Check sheet for the modelled part. Datum: model origin and axes. Units: mm. Face numbers are marked on the shaded views. A direction names the side the tool comes from. Round coordinates to 2 decimals unless told otherwise and drop trailing zeros. Order: outer loops, then holes, each group sorted by start corner. A loop starts at its lowest first (then second) coordinate and runs counter-clockwise, first axis right, second up. Notation, with made-up numbers: M 20,-37 L 33,-37 A14 cw 33,-20 Z; hole C 38.5,-5.75 d3. An arc over 180 degrees is marked long. One line per item, written item: value. Start each with the question number.
(1) Cross-section at C-C, the plane z = 20. Enter the section's corners in (x, y).
(2) Depth check by flat-ended pin: pin 1 Ø6 at (y, z) = (12, 19) entering from +X; pin 2 Ø5 at (x, y) = (31, 36.5) entering from +Z; pin 3 Ø2.5 at (x, y) = (17, -3.5) entering from -Z. Enter the tip coordinate at first touch or a pass-through.
(3) Cross-section at B-B, the plane y = 22. Enter the section's corners in (x, z), and give its area (3 significant figures).
(4) Cross-section at D-D, the plane y = 50.5. Enter the section's corners in (x, z).
(5) Thickness scan on L1, parallel to Z at x = 22.5, y = 22; L2, parallel to Y at x = 35, z = 33; L3, parallel to X at y = 7, z = 27.5. Record the ranges inside material, lowest first.
(6) Cross-section at A-A, the plane x = 31.5. Enter the section's corners in (y, z).
(7) Access from +Z, -Z, +X, -X, +Y, -Y to the whole of each face (thin tool, end or side, straight path). Record for the marked faces 1, 2 and 3.
from build123d import *

# Parameters (mm, degrees)
F0_W     = 40
F0_H     = 40
F1_DEPTH = 4
F0_H_2   = 6
F2_DEPTH = 48
F3_W     = 40
F3_H     = 3
F4_DEPTH = 5
F6_DEPTH = 3
F7_DEPTH = 20


with BuildPart() as f1:
    # F0 (on Top) → F1 (new body)
    with BuildSketch(Plane.XY):
        with Locations((20, 26)):
            Rectangle(F0_W, F0_H)
    extrude(amount=F1_DEPTH)

    # F0 (on Top) → F2 (join)
    with BuildSketch(Plane.XY):
        with Locations((20, 3)):
            Rectangle(F0_W, F0_H_2)
    extrude(amount=F2_DEPTH)

    # F3 (on face) → F4 (join)
    with BuildSketch(Plane.XZ):
        with Locations((20, 46.5)):
            Rectangle(F3_W, F3_H)
    extrude(amount=F4_DEPTH)

    # F5 (on face) → F6 (join)
    with BuildSketch(Plane(origin=(0, 0, 0), x_dir=(0, -1, 0), z_dir=(-1, 0, 0))):
        Polygon((-6, 48), (-46, 4), (-6, 4), align=None)
    extrude(amount=-F6_DEPTH)

    # F1_face (on face) → F7 (join)
    with BuildSketch(Plane(origin=(20, 46, 2), x_dir=(-1, 0, 0), z_dir=(0, 1, 0))):
        Polygon((-20, 2), (-20, -2), (20, -2), (20, 2), (17, 2), align=None)
    extrude(amount=F7_DEPTH)


solid = f1.part
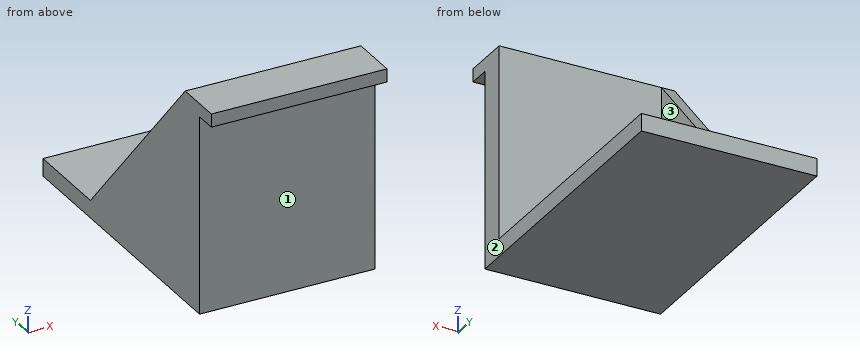
Values found:
1. outline: M 0,0 L 40,0 L 40,6 L 3,6 L 3,31.45 L 0,31.45 Z
2. pin 1: x = 3
2. pin 2: z = 4
2. pin 3: z = 45
3. outline: M 0,0 L 40,0 L 40,4 L 3,4 L 3,30.4 L 0,30.4 Z
3. area: 239 mm^2
4. outline: M 0,0 L 40,0 L 40,4 L 0,4 Z
5. L1: 0 to 4
5. L2: 0 to 6
5. L3: 0 to 3
6. outline: M -5,45 L 0,45 L 0,0 L 66,0 L 66,4 L 6,4 L 6,48 L -5,48 Z
7. face 1: -Z, +X, -X, -Y
7. face 2: +Z, -Z, +X, +Y, -Y
7. face 3: +Z, +X, +Y
